For this review, take the finished solid that the model builds, in its own axes (mm). Face numbers are marked on the shaded views. A direction names the side the tool comes from. Coordinates: 2 decimals unless noted, no trailing zeros. Write each loop counter-clockwise with the first axis right and the second up, starting at its lowest first coordinate (ties: lowest second). Pieces come first, ordered by that corner, then holes. Notation, with made-up numbers: (0.25, -21.75) -> (5.25, -21.75) arc R18 ccw to (5.25, 5.25) -> close; hole circle Ø11 at (33, -36.75). An arc over 180 degrees is marked (long way). One line per item, written item: value. Start each with the question number.
1) Mouldability with a two-part tool opening along Y and no side actions: class the marked faces 1, 2 and 3 as released by +Y, released by -Y, zero draft, split by the parting line, or undercut.
2) Machinability: for the marked faces 4, 5 and 6, which of the approach directions +Z, -Z, +X, -X, +Y, -Y give a long, thin tool a straight path to every point of the face, cutting with its end or side? Answer none if there is none.
3) Add section C-C (z = 2.3). State how many separate pieces and enclosed holes the cut face has, and give its area (3 significant figures).
4) For pin 1 Ø0.8 at (x, z) = (-7, 1.5) entering from +Y; pin 2 Ø1.6 at (y, z) = (4, 1.5) entering from +X; pin 3 Ø0.6 at (y, z) = (3.5, 1.5) entering from -X, all flat-tipped, find the tip position at first contact; note any pin that passes through.
5) Add section A-A (x = 0). State the section outline as (y, z) points, and give its area (3 significant figures).
6) Add section B-B (y = -7). State the section outline as (x, z) points.
7) For probe 1 along Y at (x, z) = (6.25, 2.35); probe 2 along X at (y, z) = (1, 1.7), list the stretches that pass through material, from the lowest coordinate up. Write a range as from..to.
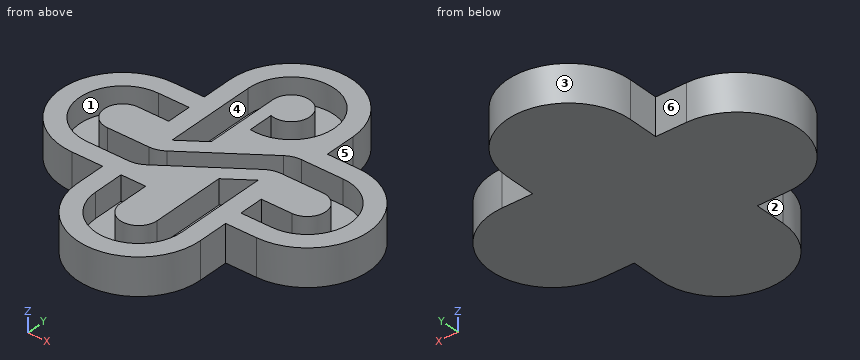
from build123d import *

# Parameters (mm, degrees)
PAD_DEPTH    = 3
POCKET_DEPTH = 2
FILLET_R     = 2
FILLET001_R  = 2
FILLET002_R  = 2
FILLET003_R  = 2


with BuildPart() as part:
    # Sketch → Pad (new body)
    with BuildSketch(Plane.XY):
        with BuildLine():
            ThreePointArc((5.000007, 7.500007), (0, 12.500023), (-5.000007, 7.500007))
            Line((-5.000007, 7.500007), (-5.000007, 5.000007))
            Line((-5.000007, 5.000007), (-7.500007, 5.000007))
            ThreePointArc((-7.500007, 5.000007), (-12.499997, 0), (-7.500007, -5.000007))
            Line((-7.500007, -5.000007), (-5.000007, -5.000007))
            Line((-5.000007, -5.000007), (-5.000007, -7.500007))
            ThreePointArc((-5.000007, -7.500007), (0, -12.500013), (5.000007, -7.500007))
            Line((5.000007, -7.500007), (5.000007, -5.000007))
            Line((5.000007, -5.000007), (7.500007, -5.000007))
            ThreePointArc((7.500007, -5.000007), (12.500003, 0), (7.500007, 5.000007))
            Line((5.000007, 5.000007), (7.500007, 5.000007))
            Line((5.000007, 7.500007), (5.000007, 5.000007))
        make_face()
    extrude(amount=PAD_DEPTH)

    # Sketch001 → Pocket (cut)
    with BuildSketch(Plane.XY.offset(3)):
        with BuildLine():
            ThreePointArc((-7.500007, 3.500007), (-10.999997, 0), (-7.500007, -3.500007))
            Line((-7.500007, -3.500007), (-3.500007, -3.500007))
            Line((-3.500007, -3.500007), (3.500007, 1.500007))
            Line((3.500007, 1.500007), (7.500007, 1.500007))
            ThreePointArc((7.499986, -1.500007), (9.000003, -1e-05), (7.500007, 1.500007))
            Line((7.499986, -1.500007), (5.000007, -1.500007))
            Line((5.000007, -1.500007), (5.000007, -3.500007))
            Line((5.000007, -3.500007), (7.499986, -3.500007))
            ThreePointArc((7.499986, -3.500007), (11.000003, -1e-05), (7.500007, 3.500007))
            Line((7.500007, 3.500007), (3.500007, 3.500007))
            Line((3.500007, 3.500007), (-3.500007, -1.500007))
            Line((-3.500007, -1.500007), (-7.500007, -1.500007))
            ThreePointArc((-7.500007, 1.500007), (-8.999997, 0), (-7.500007, -1.500007))
            Line((-7.500007, 1.500007), (-5.000007, 1.500007))
            Line((-5.000007, 3.500007), (-5.000007, 1.500007))
            Line((-7.500007, 3.500007), (-5.000007, 3.500007))
        make_face()
        with BuildLine():
            Line((-3.500007, -5.000007), (-3.500007, -7.500007))
            ThreePointArc((-3.500007, -7.500007), (0, -11.000013), (3.500007, -7.500007))
            Line((3.500007, -7.500007), (3.500007, 0))
            Line((3.500007, 0), (1.500007, -1.428573))
            Line((1.500007, -1.428573), (1.500007, -7.500007))
            ThreePointArc((-1.500007, -7.500007), (0, -9.000013), (1.500007, -7.500007))
            Line((-1.500007, -7.500007), (-1.500007, -5.000007))
            Line((-3.500007, -5.000007), (-1.500007, -5.000007))
        make_face()
        with BuildLine():
            ThreePointArc((-0.464101, 4.030917), (2.633854, 9.804981), (-3.500007, 7.50001))
            Line((-3.500007, 7.50001), (-3.500007, 0))
            Line((-3.500007, 0), (-1.500007, 1.428573))
            Line((-1.500007, 1.428573), (-1.500007, 7.500014))
            ThreePointArc((-0.464101, 6.073612), (1.213707, 8.381456), (-1.500007, 7.500014))
            Line((-0.464101, 6.073612), (-0.464101, 4.030917))
        make_face()
    extrude(amount=-POCKET_DEPTH, mode=Mode.SUBTRACT)

    # Fillet
    fillet_edges = [part.edges().sort_by_distance(p)[0] for p in [
        (3.500007, 3.500007, 2),
    ]]
    fillet(fillet_edges, radius=FILLET_R)

    # Fillet001
    fillet001_edges = [part.edges().sort_by_distance(p)[0] for p in [
        (-3.500007, -1.500007, 2),
    ]]
    fillet(fillet001_edges, radius=FILLET001_R)

    # Fillet002
    fillet002_edges = [part.edges().sort_by_distance(p)[0] for p in [
        (3.500007, 1.500007, 2),
    ]]
    fillet(fillet002_edges, radius=FILLET002_R)

    # Fillet003
    fillet003_edges = [part.edges().sort_by_distance(p)[0] for p in [
        (-3.500007, -3.500007, 2),
    ]]
    fillet(fillet003_edges, radius=FILLET003_R)


solid = part.part
Numbers:
1. face 1: undercut
1. face 2: zero draft
1. face 3: released by +Y
2. face 4: +Z
2. face 5: +Z, -Z, +X, +Y
2. face 6: +Z, -Z, -X, +Y
3. separate pieces: 1
3. enclosed holes: 3
3. area: 213 mm²
4. pin 1: y = 5
4. pin 2: x = 11.34
4. pin 3: x = -11.34
5. outline: (-12.5, 0) -> (12.5, 0) -> (12.5, 3) -> (11, 3) -> (11, 1) -> (9, 1) -> (9, 3) -> (6, 3) -> (6, 1) -> (4, 1) -> (4, 3) -> (1, 3) -> (1, 1) -> (-1, 1) -> (-1, 3) -> (-9, 3) -> (-9, 1) -> (-11, 1) -> (-11, 3) -> (-12.5, 3) -> close
5. area: 59.0 mm²
6. outline: (-5, 0) -> (5, 0) -> (5, 3) -> (3.5, 3) -> (3.5, 1) -> (1.5, 1) -> (1.5, 3) -> (-1.5, 3) -> (-1.5, 1) -> (-3.5, 1) -> (-3.5, 3) -> (-5, 3) -> close
7. probe 1: -5..-3.5, -1.5..1.5, 3.5..5
7. probe 2: -12.4..-10.85, -8.62..-3.5, -2.1..0, 2.8..8.62, 10.85..12.4
